from build123d import *

# Parameters (mm, degrees)
SKETCH1_R           = 14.75
SKETCH1_R_2         = 12
BOSS_EXTRUDE1_DEPTH = 600
SKETCH4_R           = 1.325
CUT_EXTRUDE2_DEPTH  = 10
CIRPATTERN2_COUNT   = 4
CIRPATTERN2_ANGLE   = 180
SKETCH5_R           = 13
SKETCH5_R_2         = 12
CUT_EXTRUDE3_DEPTH  = 8
LPATTERN1_COUNT     = 2
LPATTERN1_PITCH     = 592


with BuildPart() as part:
    # Sketch1 → Boss-Extrude1 (new body)
    with BuildSketch(Plane(origin=(0, 0, 0), x_dir=(1, 0, 0), z_dir=(0, 1, 0))):
        with Locations(Location((0, 0, 0), (0, 0, 270))):
            Circle(SKETCH1_R)
        with Locations(Location((0, 0, 0), (0, 0, 270))):
            Circle(SKETCH1_R_2, mode=Mode.SUBTRACT)
    extrude(amount=BOSS_EXTRUDE1_DEPTH)

    # Sketch4 → Cut-Extrude2 (cut)
    with BuildSketch(Plane.XY.offset(14.75)):
        with Locations((0, 15)):
            Circle(SKETCH4_R)
    cut_extrude2 = extrude(amount=-CUT_EXTRUDE2_DEPTH, mode=Mode.SUBTRACT)

    # CirPattern2: Cut-Extrude2 ×4 about axis
    cirpattern2_axis = Axis((0, 600, 0), (0, 1, 0))
    for i in range(1, CIRPATTERN2_COUNT):
        add(cut_extrude2.rotate(cirpattern2_axis, i * CIRPATTERN2_ANGLE / (CIRPATTERN2_COUNT - 1)), mode=Mode.SUBTRACT)

    # Sketch5 → Cut-Extrude3 (cut)
    with BuildSketch(Plane.XZ):
        with Locations(Location((0, 0, 0), (0, 0, 270))):
            Circle(SKETCH5_R)
        with Locations(Location((0, 0, 0), (0, 0, 270))):
            Circle(SKETCH5_R_2, mode=Mode.SUBTRACT)
    cut_extrude3 = extrude(amount=-CUT_EXTRUDE3_DEPTH, mode=Mode.SUBTRACT)

    # LPattern1: Cut-Extrude3 ×2
    with Locations(*[(0, i * LPATTERN1_PITCH, 0) for i in range(1, LPATTERN1_COUNT)]):
        add(cut_extrude3, mode=Mode.SUBTRACT)


solid = part.part
Work out the finished part from the listing and answer in its coordinate system (mm). A direction names the side the tool comes from. Round coordinates to 2 decimals unless told otherwise and drop trailing zeros. Write each loop counter-clockwise with the first axis right and the second up, starting at its lowest first coordinate (ties: lowest second). Pieces come first, ordered by that corner, then holes.
1) Straight lines are drawn through the part: line 1 (Y direction, x = 0, z = 13.5) (3 decimals); line 2 (Z direction, x = 0, y = 447); line 3 (X direction, y = 596.75, z = 0). For each, find the intervals that lie inside material, in ascending order.
2) The mould has two halves that part along Z. Classify faces 4 (the flat face through (-10, 600, 9)), 5 (the cylindrical face through (4.43, 295.8, 14.07)), 6 (the flat face through (-9, 8, -9)): pulls with the +Z half, pulls with the -Z half, needs draft (parallel to the pull), parting line crosses it, or undercut.
3) A cutting plane is placed at A-A (z = 0). Give the vertices of the cut face in (x, y), plus the area to 3 significant figures.
4) A tool of negligible diameter and unlimited length cuts with its end or side. For faces 1 (the flat face through (-9, 592, -9)), 2 (the cylindrical face through (3.604, 295.912, 11.446)), 3 (the cylindrical face through (-7.91, 3.944, 10.316)), from which of +Z, -Z, +X, -X, +Y, -Y can it reach the whole face along a straight path? Write none if from no direction.
5) Given pin 1 Ø8 at (x, z) = (-2, -5) entering from -Y; pin 2 Ø1.5 at (y, z) = (67.5, 1.5) entering from -X; pin 3 Ø1 at (x, y) = (-7, 419.5) entering from -Z; pin 4 Ø1.5 at (x, y) = (-8, 367.5) entering from -Z, each flat-ended and moving along its own axis, determine where each tip first touches the part or whether it passes through.
6) A cutting plane is placed at B-B (y = 407). Give the vertices of the cut face in (x, z).
Completed:
1. line 1: y = 0 to 13.675, 16.325 to 600
1. line 2: z = -14.75 to -12, 12 to 14.75
1. line 3: x = -14.75 to -13, 13 to 14.75
2. face 4: needs draft
2. face 5: parting line crosses it
2. face 6: undercut
3. outline: (-14.75, 0) - (-13, 0) - (-13, 8) - (-12, 8) - (-12, 592) - (-13, 592) - (-13, 600) - (-14.75, 600) - close; (12, 8) - (13, 8) - (13, 0) - (14.75, 0) - (14.75, 600) - (13, 600) - (13, 592) - (12, 592) - close
3. area: 3,270 mm2
4. face 1: +Y
4. face 2: +Y, -Y
4. face 3: -Y
5. pin 1: passes through
5. pin 2: stops at x = -14.73
5. pin 3: stops at z = -13.24
5. pin 4: stops at z = -12.85
6. outline: circle Ø29.5 at (0, 0); hole circle Ø24 at (0, 0)
